For this review, use the dimensioned drawing (mm, ordinates from the lowest corner) and the shaded views. A direction names the side the tool comes from. Coordinates: 2 decimals unless noted, no trailing zeros. Loops run counter-clockwise (first coordinate to the right, second up) from the corner with the lowest first, then second, coordinate; pieces in that order, holes last. Notation, with made-up numbers: M 65.25,71.5 L 94.25,71.5 A14 ccw 94.25,89.5 Z; hole C 69,75 d1. An arc over 180 degrees is marked long. Write item = value, one per line. Start each with the question number.
Q1. Wall thickness on probe 1 along X at (y, z) = (20, 20) (1 decimal); probe 2 along X at (y, z) = (6.5, 31.5); probe 3 along Y at (x, z) = (45, 20.5): over which ranges is each line inside the solid? List them lowest first.
Q2. Mouldability with a two-part tool opening along Y and no side actions: class the marked faces 3, 4 and 5 as released by +Y, released by -Y, zero draft, split by the parting line, or undercut.
Q3. Clearance check with flat-ended pins moving along their axes: pin 1 Ø2 at (x, z) = (15, 30) entering from -Y; pin 2 Ø8 at (y, z) = (7, 6.5) entering from +X; pin 3 Ø4 at (x, y) = (29.5, 20) entering from +Z. State where each tip first meets the part, or that it passes through.
Q4. We need section A-A on x = 47. Give the boundary of the cut face in (y, z), and give its area (3 significant figures).
Q5. We need section B-B on x = 31. Give the boundary of the cut face in (y, z).
Q6. We need section C-C on x = 8. Give the boundary of the cut face in (y, z) (1 decimal).
Q7. For the marked faces 1 and 2, list the 3-axis set-ups (+Z, -Z, +X, -X, +Y, -Y) from which the entire face can be reached by the end or side of a thin tool; tool diameter is ignored.
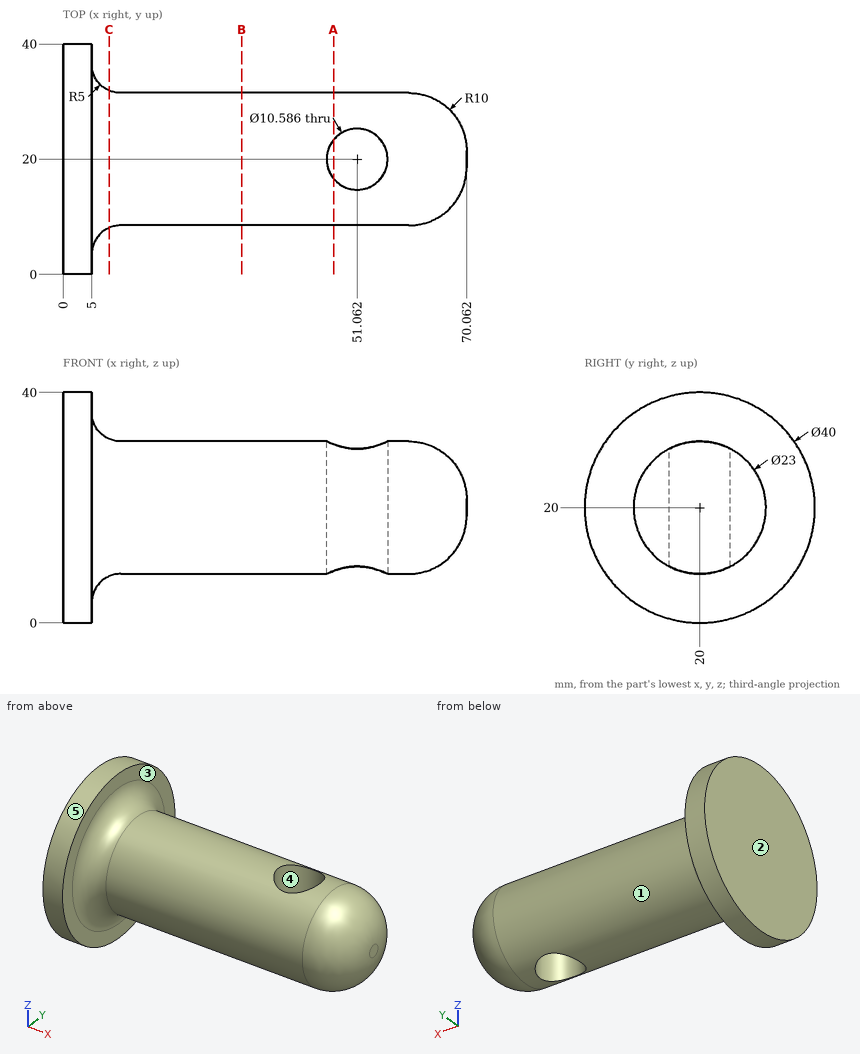
Returned:
q1.probe_1 = 0 to 45.8, 56.4 to 70.1
q1.probe_2 = 0 to 5
q1.probe_3 = 8.51 to 31.49
q2.face_3 = zero draft
q2.face_4 = undercut
q2.face_5 = split by the parting line
q3.pin_1 = 12.84
q3.pin_2 = 5.32
q3.pin_3 = 31.5
q4.outline = M 16.61,9.01 L 16.61,30.99 A11.5 ccw Z; M 23.39,9.01 A11.5 ccw 23.39,30.99 Z
q4.area = 262 mm^2
q5.outline = C 20,20 d23
q6.outline = C 20,20 d23.8
q7.face_1 = +X
q7.face_2 = +Z, -Z, -X, +Y, -Y
